Can you work these out from the model? Positions are in its coordinate system, mm. A direction names the side the tool comes from. Coordinates: 2 decimals unless noted, no trailing zeros. Order: outer loops, then holes, each group sorted by start corner. A loop starts at its lowest first (then second) coordinate and runs counter-clockwise, first axis right, second up. Notation, with made-up numbers: (56.5, 36) -> (85.5, 36) arc R9 ccw to (85.5, 53) -> close; hole circle Ø5 at (23.5, 64). An arc over 180 degrees is marked (long way). Write item = value, one per line. Start each with the question number.
from build123d import *

# Parameters (mm, degrees)
F0_W        = 21.59
F0_H        = 50.8
F1_DEPTH    = 2.54
F3_DEPTH    = 21.59
F5_DEPTH    = 21.59
F6_T1_DEPTH = 46.99
F6_T3_DEPTH = 43.18
F7_W        = 5.334
F7_H        = 5.212301854
F8_DEPTH    = 18.7325
F10_DEPTH   = 50.8
F12_DEPTH   = 21.59
F14_DEPTH   = 16.51


# Not quite as in the source:
# - a fillet or chamfer that OpenCascade refuses, or shapes differently, is made with other operations: its cross-section is extruded or revolved along the edge and cut away or added


with BuildPart() as f1:
    # F0 (on Top) → F1 (new body)
    with BuildSketch(Plane.XY):
        with Locations((10.795, 0)):
            Rectangle(F0_W, F0_H)
    extrude(amount=F1_DEPTH)

    # F2 (on Front) → F3 (cut, symmetric)
    with BuildSketch(Plane.XZ):
        with BuildLine():
            Line((19.05, 2.54), (13.716, 2.54))
            Line((13.716, 2.54), (13.3675778015, 1.2396706526))
            Line((13.3675778015, 1.2396706526), (15.0113903727, 0.7992124017))
            ThreePointArc((15.0113903727, 0.7992124017), (17.3330984682, 0.9680336444), (19.05, 2.54))
        make_face()
    extrude(amount=F3_DEPTH, both=True, mode=Mode.SUBTRACT)

    # F4 (on Front) → F5 (join, symmetric)
    with BuildSketch(Plane.XZ):
        Polygon((15.8002708221, 3.7433543202), (15.0113903727, 0.7992124017), (16.9741516517, 0.273292102), (17.7630321012, 3.2174340206), align=None)
    extrude(amount=F5_DEPTH, both=True)

    # F6: fillet of radius 0.762 on 2 edges, made by hand

    # F6_s2 → F6_t1 (cut)
    with BuildSketch(Plane.XZ.offset(-23.495)):
        with BuildLine():
            ThreePointArc((16.5363063018, 3.5461342079), (15.9580861894, 3.4700100859), (15.6030507098, 3.0073188406))
            Line((15.6030507098, 3.0073188406), (15.8002708221, 3.7433543202))
            Line((15.8002708221, 3.7433543202), (16.5363063018, 3.5461342079))
        make_face()
    extrude(amount=F6_T1_DEPTH, mode=Mode.SUBTRACT)

    # F6_s4 → F6_t3 (cut)
    with BuildSketch(Plane.XZ.offset(-21.59)):
        with BuildLine():
            ThreePointArc((17.5658119888, 2.4813985409), (17.4896878668, 3.0596186533), (17.0269966215, 3.4146541329))
            Line((17.0269966215, 3.4146541329), (17.7630321012, 3.2174340206))
            Line((17.7630321012, 3.2174340206), (17.5658119888, 2.4813985409))
        make_face()
    extrude(amount=F6_T3_DEPTH, mode=Mode.SUBTRACT)

    # F7 (on Front) → F8 (cut, symmetric)
    with BuildSketch(Plane.XZ):
        with BuildLine():
            Line((19.05, 2.54), (13.716, 2.54))
            Line((13.716, 2.54), (13.3675778015, 1.2396706526))
            Line((13.3675778015, 1.2396706526), (15.0113903727, 0.7992124017))
            ThreePointArc((15.0113903727, 0.7992124017), (17.3330984682, 0.9680336444), (19.05, 2.54))
        make_face()
        with Locations((16.383, 5.146150927)):
            Rectangle(F7_W, F7_H)
    extrude(amount=F8_DEPTH, both=True, mode=Mode.SUBTRACT)

    # F9 (on face) → F10 (join)
    with BuildSketch(Plane.XZ.offset(25.4)):
        Polygon((0, 2.54), (13.4194806689, 2.54), (2.9378255369, 5.6436832687), (0, 5.6436832687), align=None)
    extrude(amount=-F10_DEPTH)

    # F11 (on Front) → F12 (cut, symmetric)
    with BuildSketch(Plane.XZ):
        Polygon((2.4497181869, 4.1651023194), (15.0113903727, 0.7992124017), (15.0113903727, 10.927637258), (2.4497181869, 10.927637258), align=None)
    extrude(amount=F12_DEPTH, both=True, mode=Mode.SUBTRACT)

    # F13 (on Front) → F14 (join, symmetric)
    with BuildSketch(Plane.XZ):
        Polygon((12.7542149018, 1.4040207463), (13.3675778015, 1.2396706526), (13.4333178389, 1.4850158125), (12.8199549392, 1.6493659062), align=None)
    extrude(amount=F14_DEPTH, both=True)


solid = f1.part
(1) Thinking about a two-plate mould opening in X: for faces 1 (the face through (8.25, 23.47, 4.07)), 2 (the face through (17, -21.59, 3)), 3 (the face through (16, -18.732, 2)), which applies, +X half, -X half, draft (parallel to the pull), parting line (faces both ways), or undercut?
(2) If I drill on L1, parallel to Y at x = 18, z = 2.4; L2, parallel to Y at x = 15.5, z = 1.3; L3, parallel to X at y = -18, z = 4.2, over which ranges is the centre line in solid material (lowest first)? Write a range as from..to.
(3) Imagine slicing it at B-B (x = 6.25). Write out the boundary of the cut face in (y, z), plus the area to 3 significant figures.
(4) For P1, Ø2.5, axis at x = 18, y = 2.5, coming from the +Z side; P2, Ø3, axis at x = 8, y = -8, coming from the +Z side; P3, Ø0.8, axis at x = 16.5, z = 3, coming from the -Y side, each with a flat end and sliding along its axis, tell me the tip position at first contact or that it passes through.
(5) Imagine slicing it at C-C (x = 11). Write out the boundary of the cut face in (y, z).
(6) For faces 4 (the face through (8.25, -23.52, 4.07)), 5 (the face through (18, 21.59, 2)), 6 (the face through (15.31, -20.18, 1.92)), 7 (the face through (1, 0, 5.644)), 8 (the face through (17, 21.59, 3)), which set-ups out of +Z, -Z, +X, -X, +Y, -Y let a thin tool reach every point of the face, with its end or its side?
(7) Imagine slicing it at A-A (y = -10). Write out the boundary of the cut face in (x, z).
Result set:
q1.face_1 = +X half
q1.face_2 = draft
q1.face_3 = undercut
q2.L1 = -25.4..-21.59, 21.59..25.4
q2.L2 = -25.4..-18.73, 18.73..25.4
q2.L3 = 0..2.45
q3.outline = (-25.4, 0) -> (25.4, 0) -> (25.4, 4.66) -> (21.59, 4.66) -> (21.59, 3.15) -> (-21.59, 3.15) -> (-21.59, 4.66) -> (-25.4, 4.66) -> close
q3.area = 171 mm2
q4.P1 = 2.54
q4.P2 = 3.08
q4.P3 = -21.59
q5.outline = (-25.4, 0) -> (25.4, 0) -> (25.4, 3.26) -> (21.59, 3.26) -> (21.59, 1.87) -> (-21.59, 1.87) -> (-21.59, 3.26) -> (-25.4, 3.26) -> close
q6.face_4 = +Z, +X, +Y, -Y
q6.face_5 = none
q6.face_6 = +Z
q6.face_7 = +Z, +X, -X, +Y, -Y
q6.face_8 = +Z, +X, +Y
q7.outline = (0, 0) -> (21.59, 0) -> (21.59, 2.54) -> (19.05, 2.54) arc R3.55 cw to (15.01, 0.8) -> (13.37, 1.24) -> (13.43, 1.49) -> (12.82, 1.65) -> (12.75, 1.4) -> (2.45, 4.17) -> (2.45, 5.64) -> (0, 5.64) -> close
